Answer from the drawing. Dimensions are ordinates in mm from the lowest x, y and z of the part. A direction names the side the tool comes from. Round coordinates to 2 decimals unless told otherwise and drop trailing zeros. Loops run counter-clockwise (first coordinate to the right, second up) from the corner with the lowest first, then second, coordinate; pieces in that order, holes last. Notation, with made-up numbers: M 15,45 L 20,45 A27 ccw 20,61 Z; hole C 57,37.5 d9. An arc over 180 degrees is marked long. Write each question's results on one line, items separated by ' | '.
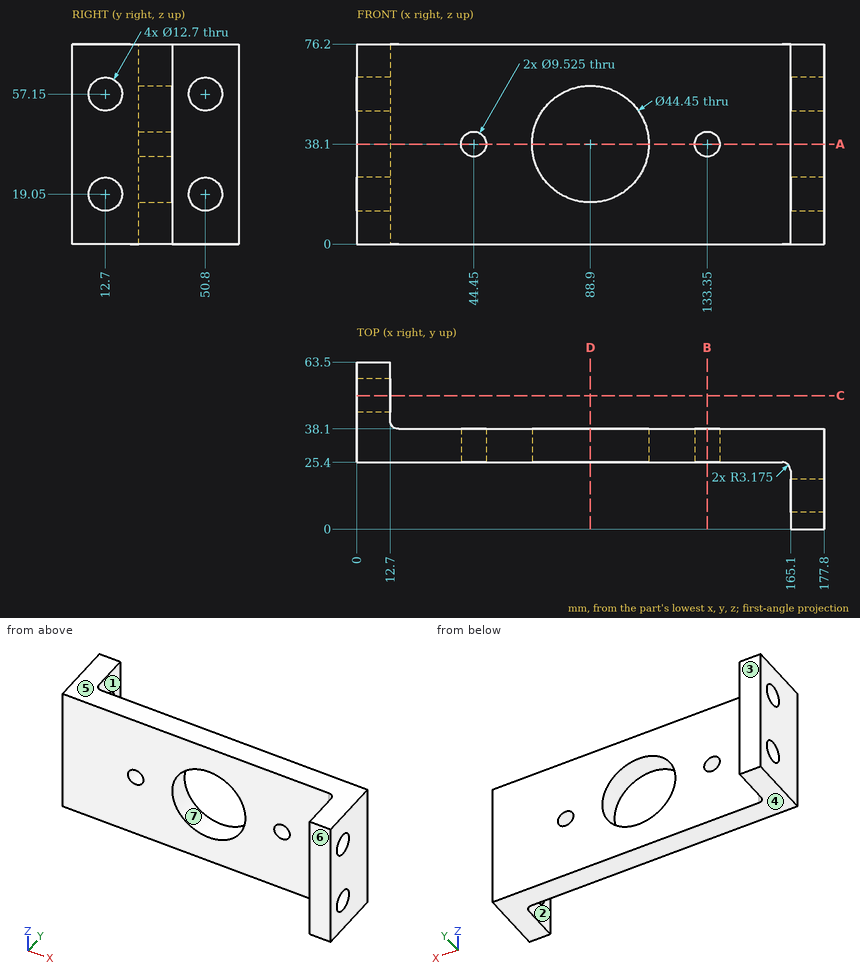
1. Find section A-A, the plane z = 38.1. Count the separate pieces of the cut face and the enclosed holes in it, then the cut area to 3 significant figures.
Completed:
separate pieces: 4 | enclosed holes: 0 | area: 2,100 mm2
2. Which of the six approach directions +Z, -Z, +X, -X, +Y, -Y give full straight-line access (tool end or side, diameter ignored) to the marked faces 1, 2 and 3?
Completed:
face 1: +Z, -Z, +X, +Y | face 2: +Z, -Z, -X, -Y | face 3: +Z, -Z, +X, -X, +Y
3. Given P1, Ø18, axis at y = 57.5, z = 22, coming from the +X side; P2, Ø18, axis at y = 16, z = 40.5, coming from the -X side; P3, Ø10, axis at x = 66.5, z = 25, coming from the +Y side, each flat-ended and moving along its own axis, determine where each tip first touches the part or whether it passes through.
Completed:
P1: stops at x = 12.7 | P2: stops at x = 163.47 | P3: stops at y = 38.1
4. Find section B-B, the plane x = 133.35. Give the vertices of the cut face in (y, z).
Completed:
outline: M 25.4,0 L 38.1,0 L 38.1,33.34 L 25.4,33.34 Z; M 25.4,42.86 L 38.1,42.86 L 38.1,76.2 L 25.4,76.2 Z
5. Find section C-C, the plane y = 50.8. Give the vertices of the cut face in (x, z), then the cut area to 3 significant figures.
Completed:
outline: M 0,0 L 12.7,0 L 12.7,12.7 L 0,12.7 Z; M 0,25.4 L 12.7,25.4 L 12.7,50.8 L 0,50.8 Z; M 0,63.5 L 12.7,63.5 L 12.7,76.2 L 0,76.2 Z | area: 645 mm2
6. Find the intervals of material crossed by L1, parallel to X at y = 34, z = 38; L2, parallel to Z at x = 6.5, y = 50.8; L3, parallel to Y at x = 174.25, z = 57.15, in increasing order.
Completed:
L1: x = 0 to 39.69, 49.21 to 66.68, 111.12 to 128.59, 138.11 to 177.8 | L2: z = 0 to 12.7, 25.4 to 50.8, 63.5 to 76.2 | L3: y = 0 to 6.35, 19.05 to 38.1
7. Find section D-D, the plane x = 88.9. Give the vertices of the cut face in (y, z) (3 decimals), then the cut area to 3 significant figures.
Completed:
outline: M 25.4,0 L 38.1,0 L 38.1,15.875 L 25.4,15.875 Z; M 25.4,60.325 L 38.1,60.325 L 38.1,76.2 L 25.4,76.2 Z | area: 403 mm2
8. Determine the mould class of the marked faces 4, 5, 6 and 7 for opening direction Z: released by +Z, released by -Z, zero draft, split by the parting line, or undercut.
Completed:
face 4: released by -Z | face 5: released by +Z | face 6: zero draft | face 7: undercut
